Source: three-view drawing plus pictorial views. Frame: mm from the lowest corner of the part. A direction names the side the tool comes from. Give positions to 0.01 mm unless a question says otherwise; leave off trailing zeros. Order: outer loops, then holes, each group sorted by start corner. A loop starts at its lowest first (then second) coordinate and runs counter-clockwise, first axis right, second up. Notation, with made-up numbers: M 65.25,57.5 L 72.25,57.5 A25 cw 72.25,81.5 Z; hole C 37.25,-31 d1. An arc over 180 degrees is marked long. Use CSV: the item, a comma, the result in double quotes.
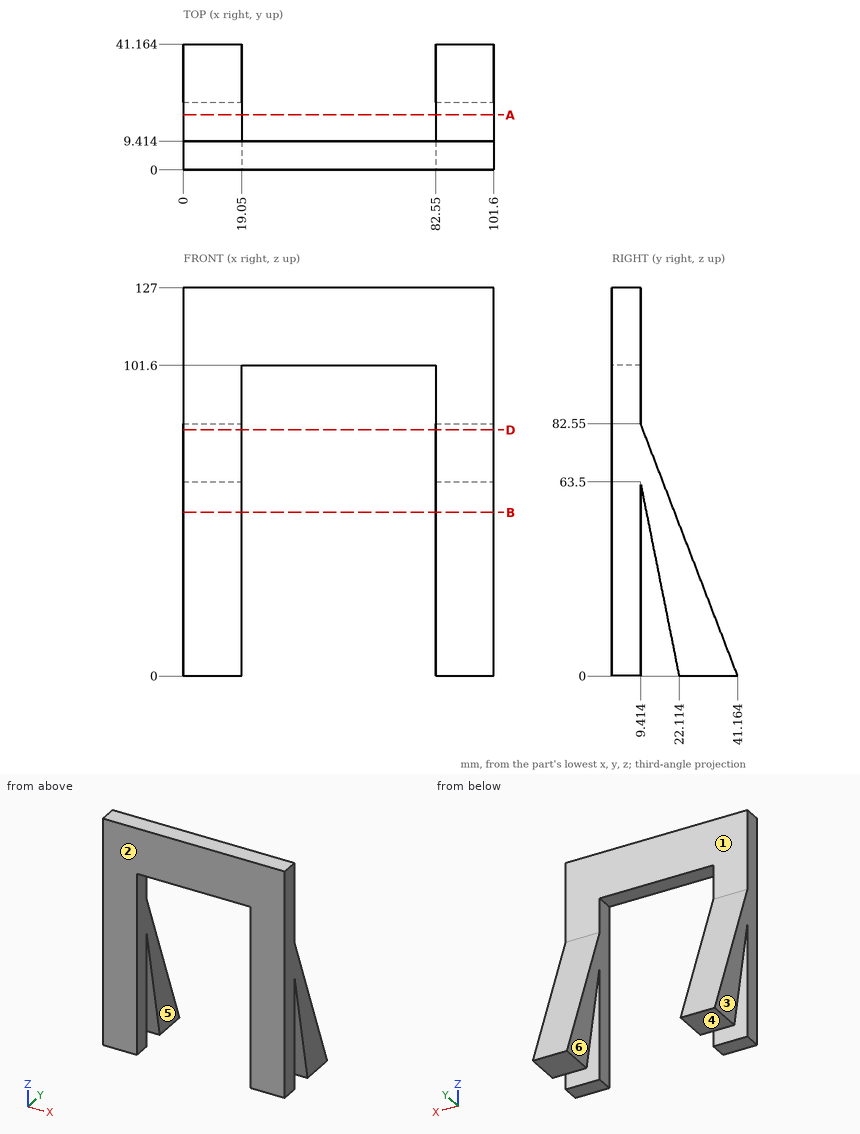
1. Line query: line 1 (X direction, y = 2.5, z = 11.5); line 2 (Y direction, x = 6, z = 21) (1 decimal); line 3 (Z direction, x = 26, y = 5.5). Output: solid intervals per line, ascending.
Answer:
line 1,"0 to 19.05, 82.55 to 101.6"
line 2,"0 to 9.4, 17.9 to 33.1"
line 3,"101.6 to 127"
2. Pull-direction query (X, two-part tool) for the marked faces 3, 4, 5 and 6; classes: +X half, -X half, draft (parallel to the pull), parting line (faces both ways), or undercut.
Answer:
face 3,"-X half"
face 4,"draft"
face 5,"undercut"
face 6,"undercut"
3. Section D-D, the plane z = 80.5. Return the cut outline in (x, y), plus the area to 3 significant figures.
Answer:
outline,"M 0,0 L 19.05,0 L 19.05,10.2 L 0,10.2 Z; M 82.55,0 L 101.6,0 L 101.6,10.2 L 82.55,10.2 Z"
area,"389 mm2"
4. Pin query (flat end, axial travel): pin 1 Ø9.5 at (x, z) = (92, 44.5) entering from +Y; pin 2 Ø21 at (x, z) = (9.5, 34) entering from +Y; pin 3 Ø3 at (x, y) = (57, 3) entering from -Z; pin 4 Ø12 at (x, y) = (19, 11.5) entering from -Z. Return the tip coordinate at first contact, or that it passes through.
Answer:
pin 1,"y = 25.88"
pin 2,"y = 32.13"
pin 3,"z = 101.6"
pin 4,"z = 0"
5. Reachability of the marked faces 1 and 2 from +Z, -Z, +X, -X, +Y, -Y: full face, straight path, thin tool, end or side. Return the list, or none.
Answer:
face 1,"+Z, +X, -X, +Y"
face 2,"+Z, -Z, +X, -X, -Y"
6. Section B-B, the plane z = 53.5. Give the number of separate pieces and of enclosed holes in the cut face, plus the area to 3 significant figures.
Answer:
separate pieces,"4"
enclosed holes,"0"
area,"708 mm2"
7. Section A-A, the plane y = 18. Return the cut outline in (x, z), plus the area to 3 significant figures.
Answer:
outline,"M 0,20.57 L 19.05,20.57 L 19.05,60.23 L 0,60.23 Z; M 82.55,20.57 L 101.6,20.57 L 101.6,60.23 L 82.55,60.23 Z"
area,"1,510 mm2"
